```python
from build123d import *

# Parameters (mm, degrees)
SKETCH1_W                = 28.575
SKETCH1_H                = 12.7
SKETCH6_R                = 3.175
BOSS_EXTRUDE1_DEPTH      = 12.7
F_1_4_20_TAPPED_HOLE1_D  = 5.1054
CIRPATTERN1_COUNT        = 4
F_10_CLEARANCE_HOLE1_D   = 5.6134
Z_0_413_DIAMETER_HOLE1_D = 10.4902


with BuildPart() as part:
    # Sketch1 → Revolve1 (revolve)
    with BuildSketch(Plane.XY, mode=Mode.PRIVATE) as revolve1_sk:
        with Locations((115.8875, 1063.625)):
            Rectangle(SKETCH1_W, SKETCH1_H)
    revolve(revolve1_sk.sketch.rotate(Axis((0, 1125.81516809, 0), (0, -1, 0)), 180), axis=Axis((0, 1125.81516809, 0), (0, -1, 0)))

    # Sketch6 → Boss-Extrude1 (add)
    with BuildSketch(Plane.XZ.offset(-1057.275)):
        with Locations(Location((-85.31243315, 85.31243315, 0), (0, 0, 180))):
            Circle(SKETCH6_R)
        with Locations(Location((85.31243315, 85.31243315, 0), (0, 0, 180))):
            Circle(SKETCH6_R)
        with Locations(Location((85.31243315, -85.31243315, 0), (0, 0, 180))):
            Circle(SKETCH6_R)
        with Locations(Location((-85.31243315, -85.31243315, 0), (0, 0, 180))):
            Circle(SKETCH6_R)
    extrude(amount=BOSS_EXTRUDE1_DEPTH)

    # 1_4-20 Tapped Hole1 (through all)
    with Locations(Plane(origin=(0, 1057.275, 0), x_dir=(-1, 0, 0), z_dir=(0, -1, 0))):
        with Locations((77.552325109, 92.423262062), (92.423262062, 77.552325109)):
            f_1_4_20_tapped_hole1 = Hole(F_1_4_20_TAPPED_HOLE1_D / 2)

    # CirPattern1: 1_4-20 Tapped Hole1 ×4 about axis
    cirpattern1_axis = Axis((0, 0, 0), (0, 1, 0))
    for i in range(1, CIRPATTERN1_COUNT):
        add(f_1_4_20_tapped_hole1.rotate(cirpattern1_axis, i * 360 / CIRPATTERN1_COUNT), mode=Mode.SUBTRACT)

    # 10 Clearance Hole1 (through all)
    with Locations(Plane(origin=(0, 1069.975, 0), x_dir=(1, 0, 0), z_dir=(0, 1, 0))):
        with Locations((112.7125, 38.1), (112.7125, 0), (112.7125, -38.1)):
            Hole(F_10_CLEARANCE_HOLE1_D / 2)

    # Z _0.413_ Diameter Hole1 (through all)
    with Locations(Plane(origin=(0, 1069.975, 0), x_dir=(1, 0, 0), z_dir=(0, 1, 0))):
        with Locations((-98.986703653, -57.15), (98.986703653, -57.15), (98.986703653, 57.15), (-98.986703653, 57.15), (-61.413345234, 96.399642256), (61.413345234, 96.399642256), (61.413345234, -96.399642256), (-61.413345234, -96.399642256)):
            Hole(Z_0_413_DIAMETER_HOLE1_D / 2)


solid = part.part
```
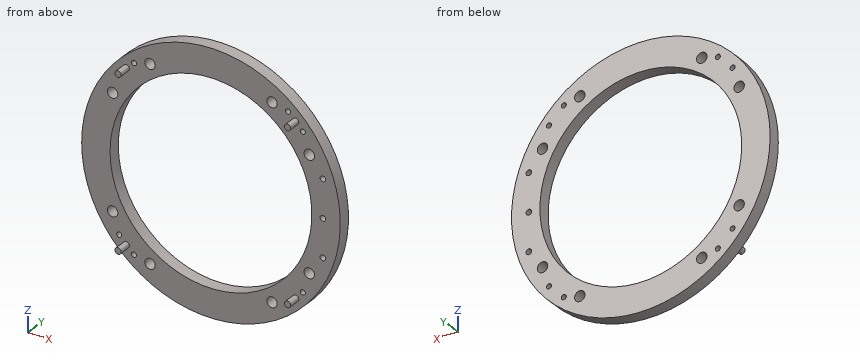
Could you check a few things on this model? Use its own coordinates, in mm. Round coordinates to 2 decimals unless told otherwise and drop trailing zeros. Write each loop counter-clockwise with the first axis right and the second up, starting at its lowest first coordinate (ties: lowest second). Pieces come first, ordered by that corner, then holes.
(1) Suppose I cut it at B-B on x = -42. Write out the boundary of the cut face in (y, z) (3 decimals), and give its area (3 significant figures).
Findings below:
outline: (1057.275, -123.213) - (1069.975, -123.213) - (1069.975, -92.512) - (1057.275, -92.512) - close; (1057.275, 92.512) - (1069.975, 92.512) - (1069.975, 123.213) - (1057.275, 123.213) - close
area: 780 mm2
(2) Suppose I cut it at C-C on y = 1063.75. State how many separate pieces and enclosed holes the cut face has, and give its area (3 significant figures).
Findings below:
separate pieces: 1
enclosed holes: 20
area: 19,900 mm2
(3) For pin 1 (13.5 mm diameter, centred on x = 61.41, z = -96.4, fed in from -Y) (3 decimals); pin 2 (9.5 mm diameter, centred on x = -98.99, z = -57.15, fed in from +Y); pin 3 (10 mm diameter, centred on y = 1051.5, z = 88.5, fed in from -X); pin 4 (8 mm diameter, centred on x = 71.5, y = 1061.5, fed in from -Z), each with a flat end and sliding along its axis, tell me the tip position at first contact or that it passes through.
Findings below:
pin 1: stops at y = 1057.275
pin 2: passes through
pin 3: stops at x = -88.49
pin 4: stops at z = -111.31
(4) Suppose I cut it at D-D on z = 57.15. Write out the boundary of the cut face in (x, y) (3 decimals).
Findings below:
outline: (-116.959, 1057.275) - (-104.232, 1057.275) - (-104.232, 1069.975) - (-116.959, 1069.975) - close; (-93.742, 1057.275) - (-84.003, 1057.275) - (-84.003, 1069.975) - (-93.742, 1069.975) - close; (84.003, 1057.275) - (93.742, 1057.275) - (93.742, 1069.975) - (84.003, 1069.975) - close; (104.232, 1057.275) - (116.959, 1057.275) - (116.959, 1069.975) - (104.232, 1069.975) - close
(5) If I drill on probe 1 along Z at (x, y) = (102.5, 1058.25); probe 2 along Y at (x, z) = (-50, -105) (3 decimals); probe 3 along X at (y, z) = (1061.5, 38.1), over which ranges is the centre line in solid material (lowest first)?
Findings below:
probe 1: z = -80.25 to -61.04, -53.26 to 53.26, 61.04 to 80.25
probe 2: y = 1057.275 to 1069.975
probe 3: x = -124.47 to -94.19, 94.19 to 109.91, 115.52 to 124.47
(6) Suppose I cut it at A-A on z = -17.5. Write out the boundary of the cut face in (x, y) (3 decimals), and give its area (3 significant figures).
Findings below:
outline: (-128.993, 1057.275) - (-100.082, 1057.275) - (-100.082, 1069.975) - (-128.993, 1069.975) - close; (100.082, 1057.275) - (128.993, 1057.275) - (128.993, 1069.975) - (100.082, 1069.975) - close
area: 734 mm2
